Autodesk Inventor part; units mm, degrees
ref_plane "YZ Plane" through (0, 0, 0) normal (1, 0, 0) x (0, 1, 0)
ref_plane "XZ Plane" through (0, 0, 0) normal (0, 1, 0) x (-1, 0, 0)
ref_plane "XY Plane" through (0, 0, 0) normal (0, 0, 1) x (1, 0, 0)
sketch "スケッチ1" plane through (0, 0, 0) normal (0, 1, 0) x (-1, 0, 0)
  line L0 (-277.5, 277.5) -> (277.5, 277.5)
  line L1 (277.5, 277.5) -> (277.5, -277.5)
  line L2 (277.5, -277.5) -> (-277.5, -277.5)
  line L3 (-277.5, -277.5) -> (-277.5, 277.5)
  line L4 (-277.5, 277.5) -> (277.5, -277.5) construction
  line L5 (277.5, 277.5) -> (-277.5, -277.5) construction
  point P0 (0, 0)
  dimension "d0" = 555
  dimension "d1" = 555
extrude "押し出し1" add sketch "スケッチ1" along normal mid plane 5
sketch "スケッチ3" plane through (0, -2.5, 0) normal (0, -1, 0) x (1, 0, 0)
  circle A0 centre (-62.5, 117.5) radius 2.5
  line L0 (277.5, -277.5) -> (277.5, 277.5)
  line L1 (-277.5, -277.5) -> (277.5, -277.5)
  circle A1 centre (-162.5, 187.5) radius 2.5
  circle A2 centre (257.5, 42.5) radius 2.5
  point P0 (0, 0)
  dimension "d10" = 5
  dimension "d15" = 5
  dimension "d16" = 320
  dimension "d17" = 20
  dimension "d18" = 5
  dimension "d24" = 75
  dimension "d25" = 320
  dimension "d26" = 420
  dimension "d27" = 145
extrude "押し出し4" cut sketch "スケッチ3" against normal through all
sketch "スケッチ5" plane through (0, -2.5, 0) normal (0, -1, 0) x (1, 0, 0)
  line L0 (277.5, 250) -> (-277.5, 250)
  line L1 (-250, 277.5) -> (-250, -277.5) construction
  line L2 (-277.5, -250) -> (277.5, -250)
  line L3 (250, -277.5) -> (250, 277.5) construction
  line L4 (-277.5, 277.5) -> (277.5, 277.5)
  line L5 (-150, 277.5) -> (277.5, 120)
  line L6 (277.5, 277.5) -> (277.5, -277.5)
  line L7 (-277.5, -277.5) -> (-277.5, 277.5)
  line L8 (-277.5, 120) -> (-150.482941, -100)
  line L9 (-150.482941, -100) -> (277.5, -100)
  line L10 (277.5, -277.5) -> (277.5, 277.5)
  point P0 (0, 0)
  dimension "d32" = 100
  dimension "d33" = 130
  dimension "d34" = 350
  dimension "d35" = 60
  dimension "d46" = 220
sketch "スケッチ5 outline for 押し出し5" plane through (0, -2.5, 0) normal (0, -1, 0) x (1, 0, 0)
  line L0 (277.5, 120) -> (277.5, 277.5)
  line L1 (-150, 277.5) -> (277.5, 120)
  line L2 (277.5, 277.5) -> (-150, 277.5)
  line L3 (-277.5, 120) -> (-277.5, -277.5)
  line L4 (-150.482941, -100) -> (-277.5, 120)
  line L5 (277.5, -100) -> (-150.482941, -100)
  line L6 (277.5, -277.5) -> (277.5, -100)
  line L7 (-277.5, -277.5) -> (277.5, -277.5)
extrude "押し出し5" cut sketch "スケッチ5 outline for 押し出し5" against normal through all
chamfer "面取り2" distance 170 distance2 100 1 edges at (-150.4829, 0, -100) measured on face at (134.839, -0.8333, -100)
sketch "スケッチ6" plane through (0, 2.5, 0) normal (0, 1, 0) x (1, 0, 0)
  line L0 (277.5, -120) -> (-150, -277.5)
  line L1 (277.5, -120) -> (277.5, -238.748566)
  line L2 (277.5, -238.748566) -> (-133.265714, -390.083302)
  line L3 (-133.265714, -390.083302) -> (-342.5, -390.083302)
  line L4 (-342.5, -390.083302) -> (-342.5, -232.583302)
  line L5 (-277.5, -277.5) -> (-277.5, -120)
  line L6 (-342.5, -232.583302) -> (-277.5, -120)
  line L7 (-200.482941, 13.39746) -> (-277.5, -120)
  line L8 (-277.5, -277.5) -> (-150, -277.5)
  point P0 (0, 0)
  dimension "d47" = 157.5
  dimension "d55" = 620
extrude "押し出し6" add sketch "スケッチ6" against normal blind 5
sketch "スケッチ7" plane through (0, 2.5, 0) normal (0, 1, 0) x (1, 0, 0)
  circle A0 centre (-242.5, -283) radius 2.5
  line L0 (277.5, -238.748566) -> (277.5, 100)
  line L1 (277.5, 100) -> (19.517059, 100)
  point P0 (0, 0)
  dimension "d50" = 5
  dimension "d51" = 520
  dimension "d52" = 383
extrude "押し出し7" cut sketch "スケッチ7" against normal through all
properties part number "endplate(flap4)"
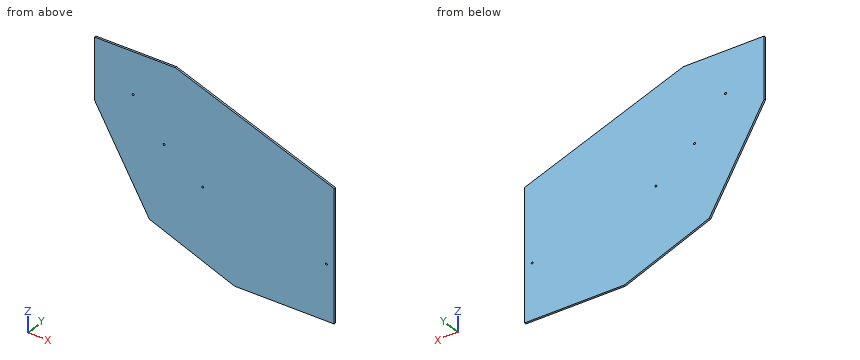
Geometry: final body of the model. Coordinates: model frame, mm. Give positions to 0.01 mm unless a question says otherwise; leave off trailing zeros. Write each loop counter-clockwise with the first axis right and the second up, starting at its lowest first coordinate (ties: lowest second). Pieces come first, ordered by that corner, then holes.
(1) First-contact query: P1, Ø3, axis at x = 108, y = -1, coming from the +Z side; P2, Ø4.5, axis at x = -62.5, z = 117.5, coming from the -Y side. Flat tips, straight axial feed; report the tip coordinate or a pass-through.
(2) Cut plane C-C, the plane z = 209. Return loops of the section in (x, y).
(3) Cut plane A-A, the plane y = -0.1. Return loops of the section in (x, z), then the cut area to 3 significant figures.
(4) Cut plane B-B, the plane x = 206. Return loops of the section in (y, z).
(5) Ray query, line 1 (Z direction, x = -242.5, y = 0.55); line 2 (Z direction, x = -62.5, y = 0.95); line 3 (X direction, y = -1.1, z = 111). Return the intervals inside material, ascending.
Values follow:
1. P1: stops at z = 301.75
1. P2: passes through
2. outline: (-328.88, -2.5) - (277.5, -2.5) - (277.5, 2.5) - (-328.88, 2.5) - close
3. outline: (-342.5, 232.58) - (-200.48, -13.4) - (19.52, -100) - (277.5, -100) - (277.5, 238.75) - (-133.27, 390.08) - (-342.5, 390.08) - close; hole circle Ø5 at (-242.5, 283); hole circle Ø5 at (-162.5, 187.5); hole circle Ø5 at (-62.5, 117.5); hole circle Ø5 at (257.5, 42.5)
3. area: 233,000 mm2
4. outline: (-2.5, -100) - (2.5, -100) - (2.5, 265.09) - (-2.5, 265.09) - close
5. line 1: z = 59.38 to 280.5, 285.5 to 390.08
5. line 2: z = -67.71 to 115, 120 to 364.01
5. line 3: x = -272.3 to 277.5
